Can you work these out from the model? Positions are in its coordinate system, mm. Face numbers are marked on the shaded views. Give positions to 0.01 mm unless a question says otherwise; leave off trailing zeros. Order: outer loops, then holes, each group sorted by start corner. A loop starts at its lowest first (then second) coordinate and runs counter-clockwise, first axis right, second up. Notation, with made-up numbers: M 71,-20.75 L 99,-20.75 A8 cw 99,-16.75 Z; hole C 52,-35.5 d10. An arc over 180 degrees is marked long. One line per question, with ' | ' between items. Start each with the question number.
1) I'm going to push a flat-ended pin straight in: pin 1 Ø9 at (x, y) = (-17.25, 20) entering from +Z. Where does the tip first touch, or does it pass through?
2) If we section it at A-A, the plane x = -41.25: Please give me the cut outline in (y, z).
3) If we section it at C-C, the plane y = -2.5: State how many separate pieces and enclosed holes the cut face has, plus the area to 3 significant figures.
4) If we section it at B-B, the plane x = 0.75: Please give me the cut outline in (y, z).
5) Thinking about a two-plate mould opening in Z: for the marked faces 1 and 2, which applies, +Z half, -Z half, draft (parallel to the pull), parting line (faces both ways), or undercut?
6) Please list where these lines run through material, in increasing order: line 1 along Y through (x, z) = (60.75, 1.4); line 2 along Y through (x, z) = (0.75, 2.5); line 3 along Y through (x, z) = (62.5, 2.55). Write a range as [from, to].
```python
from build123d import *

# Parameters (mm, degrees)
F1_DEPTH = 4
F2_R     = 4
F3_DEPTH = 4.001
F4_R     = 2


with BuildPart() as f1:
    # F0 (on Top) → F1 (new body)
    with BuildSketch(Plane.XY):
        with BuildLine():
            Line((75.25, 30), (-75.25, 30))
            Line((-75.25, 30), (-75.25, 0))
            ThreePointArc((-75.25, 0), (-72.847337, -22.262637), (-65.75, -43.5))
            Line((-65.75, -43.5), (-33.75, -43.5))
            ThreePointArc((-33.75, -43.5), (0, -21), (33.75, -43.5))
            Line((33.75, -43.5), (65.75, -43.5))
            ThreePointArc((65.75, -43.5), (72.847337, -22.262637), (75.25, 0))
            Line((75.25, 0), (75.25, 30))
        make_face()
    extrude(amount=F1_DEPTH)

    # F2 (on face) → F3 (cut, through all)
    with BuildSketch(Plane.XY.offset(4)):
        with Locations((-65.25, 20)):
            Circle(F2_R)
        with Locations((-59.25, 9.607695)):
            Circle(F2_R)
        with Locations((-53.25, 20)):
            Circle(F2_R)
        with Locations((-47.25, 9.607695)):
            Circle(F2_R)
        with Locations((-41.25, 20)):
            Circle(F2_R)
        with Locations((-35.25, 9.607695)):
            Circle(F2_R)
        with Locations((-29.25, 20)):
            Circle(F2_R)
        with Locations((-23.25, 9.607695)):
            Circle(F2_R)
        with Locations((-17.25, 20)):
            Circle(F2_R)
        with Locations((-11.25, 9.607695)):
            Circle(F2_R)
        with Locations((-5.25, 20)):
            Circle(F2_R)
        with Locations((0.75, 9.607695)):
            Circle(F2_R)
        with Locations((6.75, 20)):
            Circle(F2_R)
        with Locations((12.75, 9.607695)):
            Circle(F2_R)
        with Locations((18.75, 20)):
            Circle(F2_R)
        with Locations((24.75, 9.607695)):
            Circle(F2_R)
        with Locations((30.75, 20)):
            Circle(F2_R)
        with Locations((36.75, 9.607695)):
            Circle(F2_R)
        with Locations((42.75, 20)):
            Circle(F2_R)
        with Locations((48.75, 9.607695)):
            Circle(F2_R)
        with Locations((54.75, 20)):
            Circle(F2_R)
        with Locations((60.75, 9.607695)):
            Circle(F2_R)
        with Locations((66.75, 20)):
            Circle(F2_R)
        with Locations((-65.25, -21.569219)):
            Circle(F2_R)
        with Locations((-59.25, -31.961524)):
            Circle(F2_R)
        with Locations((-65.25, -0.78461)):
            Circle(F2_R)
        with Locations((-59.25, -11.176915)):
            Circle(F2_R)
        with Locations((-53.25, -21.569219)):
            Circle(F2_R)
        with Locations((-47.25, -31.961524)):
            Circle(F2_R)
        with Locations((-53.25, -0.78461)):
            Circle(F2_R)
        with Locations((-47.25, -11.176915)):
            Circle(F2_R)
        with Locations((-41.25, -21.569219)):
            Circle(F2_R)
        with Locations((-35.25, -31.961524)):
            Circle(F2_R)
        with Locations((-41.25, -0.78461)):
            Circle(F2_R)
        with Locations((-35.25, -11.176915)):
            Circle(F2_R)
        with Locations((-29.25, -21.569219)):
            Circle(F2_R)
        with Locations((-29.25, -0.78461)):
            Circle(F2_R)
        with Locations((-23.25, -11.176915)):
            Circle(F2_R)
        with Locations((-17.25, -0.78461)):
            Circle(F2_R)
        with Locations((-11.25, -11.176915)):
            Circle(F2_R)
        with Locations((-5.25, -0.78461)):
            Circle(F2_R)
        with Locations((0.75, -11.176915)):
            Circle(F2_R)
        with Locations((6.75, -0.78461)):
            Circle(F2_R)
        with Locations((12.75, -11.176915)):
            Circle(F2_R)
        with Locations((18.75, -0.78461)):
            Circle(F2_R)
        with Locations((24.75, -11.176915)):
            Circle(F2_R)
        with Locations((30.75, -21.569219)):
            Circle(F2_R)
        with Locations((36.75, -31.961524)):
            Circle(F2_R)
        with Locations((30.75, -0.78461)):
            Circle(F2_R)
        with Locations((36.75, -11.176915)):
            Circle(F2_R)
        with Locations((42.75, -21.569219)):
            Circle(F2_R)
        with Locations((48.75, -31.961524)):
            Circle(F2_R)
        with Locations((42.75, -0.78461)):
            Circle(F2_R)
        with Locations((48.75, -11.176915)):
            Circle(F2_R)
        with Locations((54.75, -21.569219)):
            Circle(F2_R)
        with Locations((60.75, -31.961524)):
            Circle(F2_R)
        with Locations((54.75, -0.78461)):
            Circle(F2_R)
        with Locations((60.75, -11.176915)):
            Circle(F2_R)
        with Locations((66.75, -21.569219)):
            Circle(F2_R)
        with Locations((66.75, -0.78461)):
            Circle(F2_R)
    extrude(amount=-F3_DEPTH, mode=Mode.SUBTRACT)

    # F4
    f4_edges = [f1.edges().sort_by_distance(p)[0] for p in [
        (-75.25, 30, 2),
        (-65.75, -43.5, 2),
        (-33.75, -43.5, 2),
        (33.75, -43.5, 2),
        (65.75, -43.5, 2),
        (75.25, 30, 2),
    ]]
    fillet(f4_edges, radius=F4_R)


solid = f1.part
```
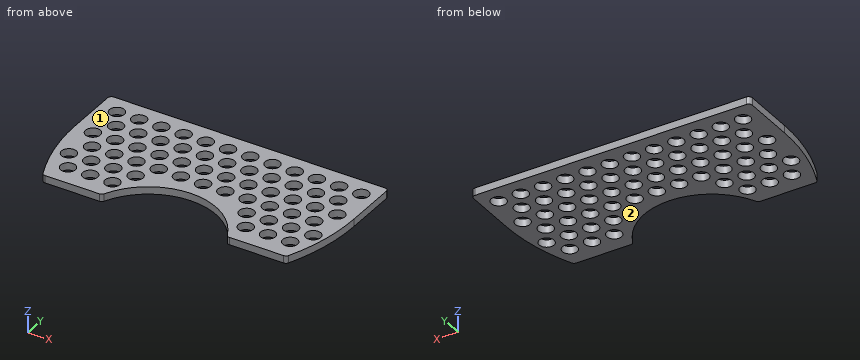
Results found:
1) pin 1: stops at z = 4
2) outline: M -43.5,0 L -25.57,0 L -25.57,4 L -43.5,4 Z; M -17.57,0 L -4.78,0 L -4.78,4 L -17.57,4 Z; M 3.22,0 L 16,0 L 16,4 L 3.22,4 Z; M 24,0 L 30,0 L 30,4 L 24,4 Z
3) separate pieces: 13 | enclosed holes: 0 | area: 255 mm²
4) outline: M -21.01,0 L -15.18,0 L -15.18,4 L -21.01,4 Z; M -7.18,0 L 5.61,0 L 5.61,4 L -7.18,4 Z; M 13.61,0 L 30,0 L 30,4 L 13.61,4 Z
5) face 1: +Z half | face 2: -Z half
6) line 1: y = [-43.5, -35.96], [-27.96, -15.18], [-7.18, 5.61], [13.61, 30] | line 2: y = [-21.01, -15.18], [-7.18, 5.61], [13.61, 30] | line 3: y = [-43.5, -35.56], [-28.36, -14.77], [-7.58, 6.01], [13.2, 30]
